from build123d import *

# Parameters (mm, degrees)
F0_W     = 25.4
F0_H     = 25.4
F0_W_2   = 23.368
F0_H_2   = 23.368
F1_DEPTH = 762
F2_R     = 2.1844
F3_DEPTH = 25.4
F4_R     = 2.1844
F5_DEPTH = 25.4


with BuildPart() as f1:
    # F0 (on Top) → F1 (new body)
    with BuildSketch(Plane.XY):
        with Locations((12.7, -12.7)):
            Rectangle(F0_W, F0_H)
        with Locations((12.7, -12.7)):
            Rectangle(F0_W_2, F0_H_2, mode=Mode.SUBTRACT)
    extrude(amount=F1_DEPTH)

    # F2 (on face) → F3 (cut)
    with BuildSketch(Plane.XZ.offset(25.4)):
        with Locations((12.7, 12.7)):
            Circle(F2_R)
        with Locations((12.7, 38.1)):
            Circle(F2_R)
        with Locations((12.7, 241.3)):
            Circle(F2_R)
        with Locations((12.7, 215.9)):
            Circle(F2_R)
        with Locations((12.7, 190.5)):
            Circle(F2_R)
        with Locations((12.7, 165.1)):
            Circle(F2_R)
        with Locations((12.7, 139.7)):
            Circle(F2_R)
        with Locations((12.7, 114.3)):
            Circle(F2_R)
        with Locations((12.7, 88.9)):
            Circle(F2_R)
        with Locations((12.7, 63.5)):
            Circle(F2_R)
        with Locations((12.7, 266.7)):
            Circle(F2_R)
        with Locations((12.7, 292.1)):
            Circle(F2_R)
        with Locations((12.7, 317.5)):
            Circle(F2_R)
        with Locations((12.7, 342.9)):
            Circle(F2_R)
        with Locations((12.7, 368.3)):
            Circle(F2_R)
        with Locations((12.7, 393.7)):
            Circle(F2_R)
        with Locations((12.7, 419.1)):
            Circle(F2_R)
        with Locations((12.7, 444.5)):
            Circle(F2_R)
        with Locations((12.7, 469.9)):
            Circle(F2_R)
        with Locations((12.7, 495.3)):
            Circle(F2_R)
        with Locations((12.7, 520.7)):
            Circle(F2_R)
        with Locations((12.7, 546.1)):
            Circle(F2_R)
        with Locations((12.7, 571.5)):
            Circle(F2_R)
        with Locations((12.7, 596.9)):
            Circle(F2_R)
        with Locations((12.7, 622.3)):
            Circle(F2_R)
        with Locations((12.7, 647.7)):
            Circle(F2_R)
        with Locations((12.7, 673.1)):
            Circle(F2_R)
        with Locations((12.7, 698.5)):
            Circle(F2_R)
        with Locations((12.7, 723.9)):
            Circle(F2_R)
        with Locations((12.7, 749.3)):
            Circle(F2_R)
    extrude(amount=-F3_DEPTH, mode=Mode.SUBTRACT)

    # F4 (on face) → F5 (cut)
    with BuildSketch(Plane(origin=(0, 0, 0), x_dir=(0, -1, 0), z_dir=(-1, 0, 0))):
        with Locations((12.7, 12.7)):
            Circle(F4_R)
        with Locations((12.7, 38.1)):
            Circle(F4_R)
        with Locations((12.7, 63.5)):
            Circle(F4_R)
        with Locations((12.7, 88.9)):
            Circle(F4_R)
        with Locations((12.7, 114.3)):
            Circle(F4_R)
        with Locations((12.7, 139.7)):
            Circle(F4_R)
        with Locations((12.7, 165.1)):
            Circle(F4_R)
        with Locations((12.7, 190.5)):
            Circle(F4_R)
        with Locations((12.7, 215.9)):
            Circle(F4_R)
        with Locations((12.7, 241.3)):
            Circle(F4_R)
        with Locations((12.7, 266.7)):
            Circle(F4_R)
        with Locations((12.7, 292.1)):
            Circle(F4_R)
        with Locations((12.7, 317.5)):
            Circle(F4_R)
        with Locations((12.7, 342.9)):
            Circle(F4_R)
        with Locations((12.7, 368.3)):
            Circle(F4_R)
        with Locations((12.7, 393.7)):
            Circle(F4_R)
        with Locations((12.7, 419.1)):
            Circle(F4_R)
        with Locations((12.7, 444.5)):
            Circle(F4_R)
        with Locations((12.7, 546.1)):
            Circle(F4_R)
        with Locations((12.7, 520.7)):
            Circle(F4_R)
        with Locations((12.7, 495.3)):
            Circle(F4_R)
        with Locations((12.7, 469.9)):
            Circle(F4_R)
        with Locations((12.7, 571.5)):
            Circle(F4_R)
        with Locations((12.7, 596.9)):
            Circle(F4_R)
        with Locations((12.7, 622.3)):
            Circle(F4_R)
        with Locations((12.7, 647.7)):
            Circle(F4_R)
        with Locations((12.7, 673.1)):
            Circle(F4_R)
        with Locations((12.7, 698.5)):
            Circle(F4_R)
        with Locations((12.7, 723.9)):
            Circle(F4_R)
        with Locations((12.7, 749.3)):
            Circle(F4_R)
    extrude(amount=-F5_DEPTH, mode=Mode.SUBTRACT)


solid = f1.part
For this review, take the finished solid that the model builds, in its own axes (mm). A direction names the side the tool comes from. Give positions to 0.01 mm unless a question says otherwise; leave off trailing zeros. Loops run counter-clockwise (first coordinate to the right, second up) from the corner with the lowest first, then second, coordinate; pieces in that order, holes last. Notation, with made-up numbers: M 43,76 L 96,76 A9 ccw 96,92 Z; hole C -9,-2.75 d11. An arc over 180 degrees is marked long. Answer as a JSON object with one key per item and string values. Group by question number.
Q1. Tool access review of faces 5 (the flat face through (13, -25.4, 376)), 6 (the flat face through (13, -24.384, 376)): name each direction out of +Z, -Z, +X, -X, +Y, -Y from which nothing blocks a thin tool from reaching the whole face with its end or side.
Q2. Mouldability with a two-part tool opening along X and no side actions: class faces 1 (the flat face through (12, -25, 0)), 2 (the flat face through (13, -1.016, 376)), 3 (the flat face through (25.4, -13, 376)), 4 (the flat face through (0, -13, 376)) as +X half, -X half, draft (parallel to the pull), parting line (faces both ways), or undercut.
Q3. Add section B-B on z = 101. Give the boundary of the cut face in (x, y).
Q4. Insertion check: P1, Ø7, axis at x = 12.7, z = 673.1, coming from the -Y side. The pin has a flat end and moves straight along its axis. Give the tip position at first contact, or say it passes through.
Q5. For probe 1 along Y at (x, z) = (14.25, 550.5); probe 2 along X at (y, z) = (-25.05, 165.1); probe 3 along X at (y, z) = (-10, 714), list the stretches that pass through material, from the lowest coordinate up. Write a range as [from, to].
Q6. Add section A-A on x = 19.25. Give the boundary of the cut face in (y, z), and give its area (3 significant figures).
Checked values:
{
 "1": {"face 5": "+Z, -Z, +X, -X, -Y", "face 6": "+Z, -Z"},
 "2": {"face 1": "draft", "face 2": "undercut", "face 3": "+X half", "face 4": "-X half"},
 "3": {"outline": "M 0,-25.4 L 25.4,-25.4 L 25.4,0 L 0,0 Z; hole M 1.02,-24.38 L 24.38,-24.38 L 24.38,-1.02 L 1.02,-1.02 Z"},
 "4": {"P1": "y = -25.4"},
 "5": {"probe 1": "[-25.4, -24.38], [-1.02, 0]", "probe 2": "[0, 10.52], [14.88, 25.4]", "probe 3": "[0, 1.02], [24.38, 25.4]"},
 "6": {"outline": "M -25.4,0 L -24.38,0 L -24.38,762 L -25.4,762 Z; M -1.02,0 L 0,0 L 0,762 L -1.02,762 Z", "area": "1,550 mm²"}
}
